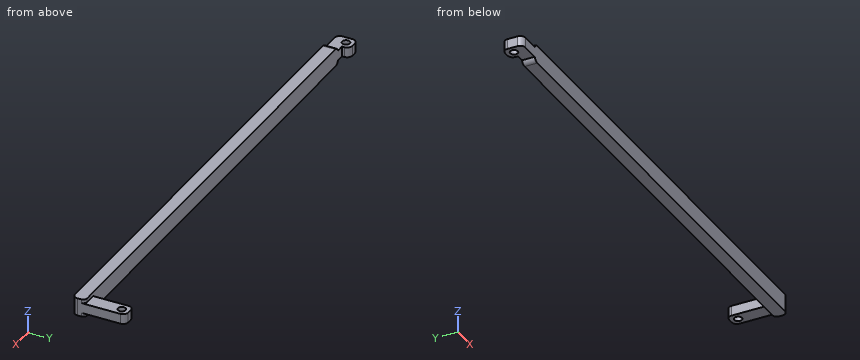
Autodesk Inventor part; units mm, degrees
ref_plane "YZ Plane" through (0, 0, 0) normal (1, 0, 0) x (0, 1, 0)
ref_plane "XZ Plane" through (0, 0, 0) normal (0, 1, 0) x (-1, 0, 0)
ref_plane "XY Plane" through (0, 0, 0) normal (0, 0, 1) x (1, 0, 0)
sketch "Sketch1" plane through (0, 0, 0) normal (0, 1, 0) x (-1, 0, 0)
  line L0 (99.05, 3.5) -> (-99.05, 3.5)
  line L1 (-99.05, 3.5) -> (-99.05, -3.5)
  line L2 (-99.05, -3.5) -> (99.05, -3.5)
  line L3 (99.05, -3.5) -> (99.05, 3.5)
  line L4 (99.05, 3.5) -> (-99.05, -3.5) construction
  line L5 (-99.05, 3.5) -> (99.05, -3.5) construction
  point P0 (0, 0)
  dimension "d0" = 198.1
  dimension "d1" = 7
extrude "Extrusion1" add sketch "Sketch1" along normal blind 5
sketch "Sketch2" plane through (0, 5, 0) normal (0, 1, 0) x (1, 0, 0)
  line L0 (99.05, -3.5) -> (99.05, 3.5)
  line L1 (99.05, 2) -> (93.05, 2)
  line L2 (93.05, 2) -> (93.05, -2)
  line L3 (93.05, -2) -> (99.05, -2)
  line L4 (99.05, -2) -> (99.05, 2)
  line L5 (99.05, 3.5) -> (-99.05, 3.5)
  point P0 (0, 0)
  dimension "d25" = 6
  dimension "d26" = 4
  dimension "d27" = 1.5
extrude "Extrusion2" add sketch "Sketch2" along normal blind 15.875
fillet "Fillet1" radius 2 2 edges at (99.05, 20.875, 0) (93.05, 20.875, 0)
sketch "Sketch4" plane through (0, 5, 0) normal (0, 1, 0) x (1, 0, 0)
  line L0 (99.05, 3.5) -> (-99.05, 3.5)
  line L1 (-99.05, 2) -> (-93.05, 2)
  line L2 (-93.05, 2) -> (-93.05, -2)
  line L3 (-93.05, -2) -> (-99.05, -2)
  line L4 (-99.05, -2) -> (-99.05, 2)
  line L5 (-99.05, 3.5) -> (-99.05, -3.5)
  point P0 (0, 0)
  dimension "d33" = 6
  dimension "d34" = 4
  dimension "d35" = 6
  dimension "d36" = 1.5
extrude "Extrusion4" add sketch "Sketch4" along normal blind 3
fillet "Fillet2" radius 2 2 edges at (-93.05, 8, 0) (-99.05, 8, 0)
fillet "Fillet3" radius 2 2 edges at (99.05, 0, 0) (-99.05, 0, 0)
sketch "Sketch6" plane through (93.05, 5, 2) normal (0, 0, 1) x (1, 0, 0)
  line L0 (0, 15.875) -> (6, 15.875) construction
  line L1 (3, 15.875) -> (3, 12.875) construction
  line L2 (3, 15.875) -> (6, 15.875) construction
  circle A0 centre (3, 12.875) radius 1.5
  point P0 (-93.05, -5)
  dimension "d28" = 3
  dimension "d29" = 90
  dimension "d30" = 3
extrude "Extrusion6" cut sketch "Sketch6" against normal through all
sketch "Sketch7" plane through (-99.05, 5, 2) normal (0, 0, 1) x (1, 0, 0)
  line L0 (4, 3) -> (2, 3) construction
  line L1 (3, 3) -> (3, 0) construction
  line L2 (3, 3) -> (6, 3) construction
  circle A0 centre (3, 0) radius 1.5
  point P0 (99.05, -5)
  dimension "d57" = 1.5
  dimension "d37" = 3
  dimension "d38" = 90
  dimension "d39" = 3
sketch "Sketch8" plane through (0, 5, 0) normal (0, 1, 0) x (1, 0, 0)
  line L0 (-99.05, -3.5) -> (99.05, -3.5)
  line L1 (-93.05, -2) -> (-99.05, -2)
  line L2 (-99.05, -2) -> (-90.05, -2)
  line L3 (-90.05, -2) -> (-90.05, -3.5)
  line L4 (-90.05, -3.5) -> (-99.05, -3.5)
  line L5 (-99.05, -3.5) -> (-99.05, -2)
  line L6 (-99.05, 3.5) -> (-90.05, 3.5)
  line L7 (-90.05, 3.5) -> (-90.05, 2)
  line L8 (-90.05, 2) -> (-99.05, 2)
  line L9 (-99.05, 2) -> (-99.05, 3.5)
  point P0 (0, 0)
  dimension "d54" = 9
  dimension "d55" = 1.5
  dimension "d56" = 9
  dimension "d57" = 1.5
extrude "Extrusion7" cut sketch "Sketch8" against normal through all
extrude "Extrusion8" cut sketch "Sketch7" against normal through all
fillet "Fillet5" radius 1.5 2 edges at (99.05, 5, 2.75) (99.05, 5, -2.75)
fillet "Fillet6" radius 2 2 edges at (-90.05, 2.5, 3.5) (-90.05, 2.5, -3.5)
properties part number "Brace_unequal"
Geometry check sheet. Reference: the model listing, model coordinates, mm. Coordinates: 2 decimals unless noted, no trailing zeros. Order: outer loops, then holes, each group sorted by start corner. A loop starts at its lowest first (then second) coordinate and runs counter-clockwise, first axis right, second up.
Q1. Thickness scan on probe 1 along Y at (x, z) = (-96.05, -0.8); probe 2 along Y at (x, z) = (96.05, -0.35) (3 decimals); probe 3 along X at (y, z) = (14, 0). Record the ranges inside material, lowest first.
Reply:
probe 1: y = 0 to 3.5, 6.5 to 8
probe 2: y = 0 to 16.375, 19.375 to 20.875
probe 3: x = 93.05 to 99.05
Q2. Depth check by flat-ended pin: pin 1 Ø0.6 at (x, z) = (-95.5, 0) entering from +Y; pin 2 Ø3 at (y, z) = (14, -1) entering from -X; pin 3 Ø1 at (x, z) = (49.5, 2.5) entering from -Y; pin 4 Ø3 at (x, z) = (-23.5, 1) entering from +Y. Enter the tip coordinate at first touch or a pass-through.
Reply:
pin 1: stops at y = 8
pin 2: stops at x = 93.05
pin 3: stops at y = 0
pin 4: stops at y = 5
Q3. Sectioned sample at B-B on y = 10.25. Record the cut outline in (x, z).
Reply:
outline: (93.05, -2) - (99.05, -2) - (99.05, 2) - (93.05, 2) - close
Q4. Sectioned sample at C-C on x = -41.5. Record the cut outline in (y, z), and give its area (3 significant figures).
Reply:
outline: (0, -3.5) - (5, -3.5) - (5, 3.5) - (0, 3.5) - close
area: 35.0 mm2
Q5. Sectioned sample at A-A on z = 0. Record the cut outline in (x, y) (3 decimals), and give its area (3 significant figures).
Reply:
outline: (-99.05, 2) arc R2 ccw to (-97.05, 0) - (97.05, 0) arc R2 ccw to (99.05, 2) - (99.05, 18.875) arc R2 ccw to (97.05, 20.875) - (95.05, 20.875) arc R2 ccw to (93.05, 18.875) - (93.05, 5) - (-93.05, 5) - (-93.05, 6) arc R2 ccw to (-95.05, 8) - (-97.05, 8) arc R2 ccw to (-99.05, 6) - close; hole circle Ø3 at (-96.05, 5); hole circle Ø3 at (96.05, 17.875)
area: 1,080 mm2
